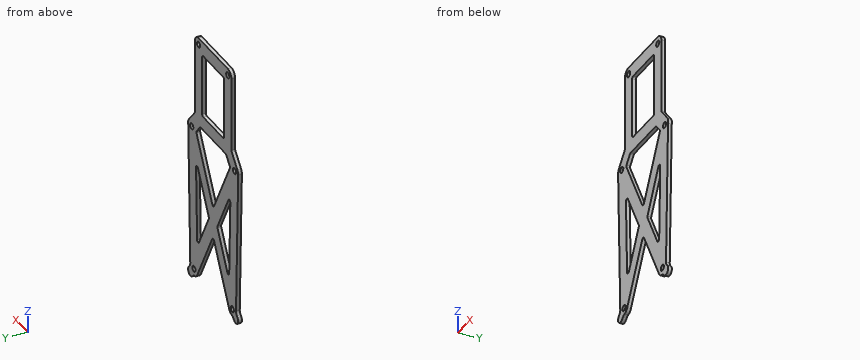
Autodesk Inventor part; units mm, degrees
ref_plane "YZ Plane" through (0, 0, 0) normal (1, 0, 0) x (0, 1, 0)
ref_plane "XZ Plane" through (0, 0, 0) normal (0, 1, 0) x (-1, 0, 0)
ref_plane "XY Plane" through (0, 0, 0) normal (0, 0, 1) x (1, 0, 0)
sketch "Szkic1" plane through (0, 0, 0) normal (0, 1, 0) x (-1, 0, 0)
  line L0 (-14.9332, 17.4281) -> (15.0668, 17.4281) construction
  line L1 (-14.9332, 13.6781) -> (15.0668, 13.6781)
  line L2 (15.0668, 21.1781) -> (-14.9332, 21.1781)
  arc A0 (-14.9332, 21.1781) -> (-14.9332, 13.6781) centre (-14.9332, 17.4281) ccw
  arc A1 (15.0668, 13.6781) -> (15.0668, 21.1781) centre (15.0668, 17.4281) ccw
  line L3 (0.0668, 17.4281) -> (0.0668, -37.9617) construction
  line L4 (15.0668, 17.4281) -> (15.0668, -55.6314) construction
  line L5 (-14.9332, 17.4281) -> (-14.9332, -55.6314) construction
  line L6 (22.0668, -33.0639) -> (15.0668, -24.7796) construction
  line L7 (24.9311, -30.6436) -> (17.9311, -22.3593)
  line L8 (12.2024, -27.1999) -> (19.2024, -35.4842)
  arc A2 (19.2024, -35.4842) -> (24.9311, -30.6436) centre (22.0668, -33.0639) ccw
  arc A3 (17.9311, -22.3593) -> (12.2024, -27.1999) centre (15.0668, -24.7796) ccw
  line L9 (-21.9332, -33.0639) -> (-14.9332, -24.7796) construction
  line L10 (-19.0689, -35.4842) -> (-12.0689, -27.1999)
  line L11 (-17.7976, -22.3593) -> (-24.7976, -30.6436)
  arc A4 (-24.7976, -30.6436) -> (-19.0689, -35.4842) centre (-21.9332, -33.0639) ccw
  arc A5 (-12.0689, -27.1999) -> (-17.7976, -22.3593) centre (-14.9332, -24.7796) ccw
  line L12 (15.0668, 17.4281) -> (15.0668, -24.7796) construction
  line L13 (11.3168, 17.4281) -> (11.3168, -24.7796)
  line L14 (18.8168, -24.7796) -> (18.8168, 17.4281)
  arc A6 (18.8168, 17.4281) -> (11.3168, 17.4281) centre (15.0668, 17.4281) ccw
  arc A7 (11.3168, -24.7796) -> (18.8168, -24.7796) centre (15.0668, -24.7796) ccw
  line L15 (-14.9332, 17.4281) -> (-14.9332, -24.7796) construction
  line L16 (-18.6832, 17.4281) -> (-18.6832, -24.7796)
  line L17 (-11.1832, -24.7796) -> (-11.1832, 17.4281)
  arc A8 (-11.1832, 17.4281) -> (-18.6832, 17.4281) centre (-14.9332, 17.4281) ccw
  arc A9 (-18.6832, -24.7796) -> (-11.1832, -24.7796) centre (-14.9332, -24.7796) ccw
  line L18 (-14.9332, -24.7796) -> (15.0668, -24.7796) construction
  line L19 (-14.9332, -21.0296) -> (15.0668, -21.0296)
  line L20 (15.0668, -28.5296) -> (-14.9332, -28.5296)
  arc A10 (-14.9332, -21.0296) -> (-14.9332, -28.5296) centre (-14.9332, -24.7796) ccw
  arc A11 (15.0668, -28.5296) -> (15.0668, -21.0296) centre (15.0668, -24.7796) ccw
  line L21 (22.0668, -33.0639) -> (19.8168, -113.0323) construction
  line L22 (18.3183, -32.9584) -> (16.0683, -112.9268)
  line L23 (23.5653, -113.1377) -> (25.8153, -33.1694)
  arc A12 (25.8153, -33.1694) -> (18.3183, -32.9584) centre (22.0668, -33.0639) ccw
  arc A13 (16.0683, -112.9268) -> (23.5653, -113.1377) centre (19.8168, -113.0323) ccw
  line L24 (-21.8084, -33.1694) -> (-19.6832, -113.0323) construction
  line L25 (-25.5571, -33.2691) -> (-23.4319, -113.132)
  line L26 (-15.9346, -112.9325) -> (-18.0597, -33.0696)
  arc A14 (-18.0597, -33.0696) -> (-25.5571, -33.2691) centre (-21.8084, -33.1694) ccw
  arc A15 (-23.4319, -113.132) -> (-15.9346, -112.9325) centre (-19.6832, -113.0323) ccw
  line L27 (22.0668, -33.0639) -> (-19.6832, -113.0323) construction
  line L28 (18.7425, -31.3284) -> (-23.0075, -111.2967)
  line L29 (-16.359, -114.7678) -> (25.391, -34.7994)
  arc A16 (25.391, -34.7994) -> (18.7425, -31.3284) centre (22.0668, -33.0639) ccw
  arc A17 (-23.0075, -111.2967) -> (-16.359, -114.7678) centre (-19.6832, -113.0323) ccw
  line L30 (-21.8084, -33.1694) -> (19.8168, -113.0323) construction
  line L31 (-25.1338, -34.9026) -> (16.4914, -114.7655)
  line L32 (23.1422, -111.299) -> (-18.483, -31.4361)
  arc A18 (-18.483, -31.4361) -> (-25.1338, -34.9026) centre (-21.8084, -33.1694) ccw
  arc A19 (16.4914, -114.7655) -> (23.1422, -111.299) centre (19.8168, -113.0323) ccw
  point P0 (0, 0)
  point P1 (18.5668, -28.9217)
  point P2 (-18.4332, -28.9217)
  point P3 (15.0668, -3.6757)
  point P4 (-14.9332, -3.6757)
  point P5 (0.0668, -24.7796)
  point P6 (20.9418, -73.0481)
  point P7 (-20.7458, -73.1008)
  point P8 (1.1918, -73.0481)
  point P9 (-0.9958, -73.1008)
  point P10 (-18.6832, -23.4074)
  point P11 (-25.5347, -34.1087)
  point P12 (0.0805, -83.2794)
  point P13 (24.9311, -30.6436)
  point P14 (18.8168, -23.4074)
  point P15 (4.3129, -75.1727)
  point P16 (17.8606, -49.2232)
  point P17 (16.474, -98.5053)
  point P18 (-4.1462, -75.1698)
  point P19 (-16.319, -98.4856)
  point P20 (-17.6277, -49.3039)
  point P21 (0.0861, -67.0631)
  point P22 (-17.4016, -33.511)
  point P23 (-13.1924, -28.5296)
  point P24 (13.3259, -28.5296)
  point P25 (17.5771, -33.5607)
  point P26 (11.3168, 13.6781)
  point P27 (11.3168, -21.0296)
  point P28 (-11.1832, -21.0296)
  point P29 (-11.1832, 13.6781)
  dimension "d0" = 7.5
  dimension "d1" = 7.5
  dimension "d2" = 7.5
  dimension "d3" = 7.5
  dimension "d4" = 7.5
  dimension "d5" = 7.5
  dimension "d6" = 7.5
extrude "Wyciągnięcie proste1" add sketch "Szkic1" along normal blind 2 contours A0 A8 L17 L1 | L1 L17 L19 A5 L11 L16 A0 | L17 A8 L2 A6 L13 L1 | L13 A6 A1 L1 | L1 A1 L14 L7 A3 L19 L13 | L19 L13 A3 L8 L20 L10 A5 L17 | L17 A5 L19 | L16 A9 L20 L10 L32 A14 L25 A4 L11 | L11 A10 L16 | L19 A3 L13 | A5 A9 A10 | A3 A11 A7 | L10 L20 A9 | L25 A18 L31 A4 | A4 L31 L26 L28 A17 L25 | L14 A11 L7 | L7 A12 L28 L8 L20 A7 L14 | A7 L20 L8 | L31 A18 A14 L26 L10 A4 | A4 L10 L26 L31 | A17 L28 L26 A15 | A2 L8 L22 A12 | L32 L28 L31 L26 L10 | L10 L26 A14 L32 | A15 L26 L28 L31 L29 | L23 A19 L32 L22 L29 A2 | A12 L22 L8 L28 | L8 L22 L29 L32 L28 | L32 L29 L31 L28 | L29 L32 L22 A13 L31 | L29 L22 L8 A2 | A13 L22 L32 A19
fillet "Zaokrąglenie1" radius 1 18 edges at (-0.0805, 1, -83.2794) (-4.3129, 1, -75.1727) (4.1462, 1, -75.1698) (-0.0861, 1, -67.0631) (-17.8606, 1, -49.2232) (-16.474, 1, -98.5053) (16.319, 1, -98.4856) (17.6277, 1, -49.3039) (17.4016, 1, -33.511) (13.1924, 1, -28.5296) (-18.8168, 1, -23.4074) (-17.5771, 1, -33.5607) (-13.3259, 1, -28.5296) (-11.3168, 1, -21.0296) (11.1832, 1, -21.0296) (11.1832, 1, 13.6781) (-11.3168, 1, 13.6781) (18.6832, 1, -23.4074)
sketch "Szkic5" plane through (0, 0, 0) normal (0, -1, 0) x (1, 0, 0)
  arc A0 (18.6832, 17.4281) -> (14.9332, 21.1781) centre (14.9332, 17.4281) ccw
  arc A1 (-15.0668, 21.1781) -> (-18.8168, 17.4281) centre (-15.0668, 17.4281) ccw
  arc A2 (25.5347, -34.1087) -> (24.7976, -30.6436) centre (21.9332, -33.0639) ccw
  arc A3 (-24.9311, -30.6436) -> (-25.8153, -33.1694) centre (-22.0668, -33.0639) ccw
  arc A4 (16.359, -114.7678) -> (23.4319, -113.132) centre (19.6832, -113.0323) ccw
  arc A5 (-23.5653, -113.1377) -> (-16.4914, -114.7655) centre (-19.8168, -113.0323) ccw
  point P0 (0, 0)
hole "Otwór2" at (21.9332, 0, -33.0639) at (-22.0668, 0, -33.0639) at (14.9332, 0, 17.4281) at (-15.0668, 0, 17.4281) at (19.6832, 0, -113.0323) at (-19.8168, 0, -113.0323) direction (0, 1, 0) diameter 3.2 depth 6
sketch "Szkic6" plane through (0, 0, 0) normal (0, -1, 0) x (1, 0, 0)
  circle A0 centre (19.6832, -113.0323) radius 1.6
  circle A1 centre (-19.8168, -113.0323) radius 1.6
  line L0 (19.6832, -113.0323) -> (23.2188, -116.5678) construction
  line L1 (17.9155, -114.8) -> (21.451, -118.3356)
  line L2 (24.9865, -114.8) -> (21.451, -111.2645)
  arc A2 (21.451, -111.2645) -> (17.9155, -114.8) centre (19.6832, -113.0323) ccw
  arc A3 (21.451, -118.3356) -> (24.9865, -114.8) centre (23.2188, -116.5678) ccw
  line L3 (-19.8168, -113.0323) -> (-23.3523, -116.5678) construction
  line L4 (-21.5845, -111.2645) -> (-25.1201, -114.8)
  line L5 (-21.5845, -118.3356) -> (-18.049, -114.8)
  arc A4 (-18.049, -114.8) -> (-21.5845, -111.2645) centre (-19.8168, -113.0323) ccw
  arc A5 (-25.1201, -114.8) -> (-21.5845, -118.3356) centre (-23.3523, -116.5678) ccw
  line L6 (12.7282, -28.5296) -> (-12.8617, -28.5296)
  point P0 (0, 0)
  point P1 (21.451, -114.8)
  point P2 (-21.5845, -114.8)
  dimension "d29" = 5
  dimension "d30" = 5
  dimension "d31" = 5
  dimension "d32" = 5
  dimension "d33" = 45
extrude "Wyciągnięcie proste3" add sketch "Szkic6" against normal blind 2
fillet "Zaokrąglenie3" radius 3 4 edges at (19.8919, 1, -116.7764) (23.4274, 1, -113.2409) (-20.0254, 1, -116.7764) (-23.561, 1, -113.2409)
properties part number "mocowanie"
Here's how the part is built. I have some questions about the finished solid (model axes, mm). Round coordinates to 2 decimals unless told otherwise and drop trailing zeros. Order: outer loops, then holes, each group sorted by start corner. A loop starts at its lowest first (then second) coordinate and runs counter-clockwise, first axis right, second up. Notation, with made-up numbers: (50, 5) -> (101, 5) arc R14 cw to (101, 18) -> close; hole circle Ø7 at (-23, -3.5). An arc over 180 degrees is marked (long way). Use a Markdown table: item, result. Add a question column.
(1) For pin 1 Ø1.9 at (x, z) = (-22.07, -33.06) entering from +Y; pin 2 Ø1 at (x, y) = (3.5, 0.5) entering from -Z; pin 3 Ø1 at (x, y) = (-14, 1.5) entering from -Z; pin 4 Ø1 at (x, y) = (-1.5, 1) entering from -Z, each with a flat end and sliding along its axis, tell me the tip position at first contact or that it passes through.
(2) Suppose I cut it at B-B, the plane z = -58. Please give me the cut outline in (x, y), and give its area (3 significant figures).
(3) Suppose I cut it at A-A, the plane z = 1. Please give me the cut outline in (x, y).
(4) I need wall thicknesses on line 1 along X through (y, z) = (0.35, -1); line 2 along Z through (x, y) = (-12.5, 1.85); line 3 along X through (y, z) = (1.6, -68). Which ranges of each line are inside material? Lowest first, please.
(5) Suppose I cut it at C-C, the plane y = 0.6. Count the separate pieces of the cut face and the enclosed holes in it, and give its area (3 significant figures).
Verdict:
| question | item | result |
|---|---|---|
| 1 | pin 1 | through |
| 1 | pin 2 | z = -91.1 |
| 1 | pin 3 | z = -110.94 |
| 1 | pin 4 | z = -86.96 |
| 2 | outline | (-25.12, 0) -> (-17.61, 0) -> (-17.61, 2) -> (-25.12, 2) -> close; (-13.28, 0) -> (-4.82, 0) -> (-4.82, 2) -> (-13.28, 2) -> close; (4.64, 0) -> (13.1, 0) -> (13.1, 2) -> (4.64, 2) -> close; (17.4, 0) -> (24.9, 0) -> (24.9, 2) -> (17.4, 2) -> close |
| 2 | area | 63.8 mm2 |
| 3 | outline | (-18.82, 0) -> (-11.32, 0) -> (-11.32, 2) -> (-18.82, 2) -> close; (11.18, 0) -> (18.68, 0) -> (18.68, 2) -> (11.18, 2) -> close |
| 4 | line 1 | -18.82 to -11.32, 11.18 to 18.68 |
| 4 | line 2 | -107.11 to -90.88, -59.49 to -43.29, -28.53 to 21.18 |
| 4 | line 3 | -24.84 to -17.33, -8.06 to 7.88, 17.13 to 24.63 |
| 5 | separate pieces | 1 |
| 5 | enclosed holes | 10 |
| 5 | area | 3,470 mm2 |
